Autodesk Fusion 360 part; units mm, degrees
sketch "Sketch1" plane through (0, 0, 0) normal (0, 1, 0) x (1, 0, 0)
  line L0 (7.5, -22.5) -> (-7.5, -22.5)
  line L1 (-7.5, -22.5) -> (-7.5, 22.5)
  line L2 (-7.5, 22.5) -> (7.5, 22.5)
  line L3 (7.5, 22.5) -> (7.5, -22.5)
  line L4 (7.5, -22.5) -> (-7.5, 22.5) construction
  line L5 (-7.5, -22.5) -> (7.5, 22.5) construction
  dimension "d1" = 45
  dimension "d2" = 15
extrude "Extrude1" add sketch "Sketch1" along normal blind 4
sketch "Sketch2" plane through (0, 4, 0) normal (0, 1, 0) x (-1, 0, 0)
  line L0 (-7.5, -22.5) -> (7.5, -22.5)
  line L1 (7.5, -22.5) -> (7.5, 22.5)
  line L2 (7.5, 22.5) -> (-7.5, 22.5)
  line L3 (-7.5, 22.5) -> (-7.5, -22.5)
  line L4 (-7.5, 22.5) -> (-3.5, 22.5)
  line L5 (-3.5, 22.5) -> (-3.5, -22.5)
  line L6 (-3.5, -22.5) -> (-7.5, -22.5)
  line L7 (-7.5, -22.5) -> (-7.5, 22.5)
  dimension "d9" = 4
extrude "Extrude2" add sketch "Sketch2" along normal blind 64 contours L0 L2 L3 L4 L5 L6 L7
sketch "Sketch3" plane through (3.5, 0, 0) normal (-1, 0, 0) x (0, -1, 0)
  line L0 (-4, -22.5) -> (-4, 22.5)
  line L1 (-4, 22.5) -> (-68, 22.5)
  line L2 (-68, 22.5) -> (-68, -22.5)
  line L3 (-68, -22.5) -> (-4, -22.5)
  line L4 (-68, 22.5) -> (-64, 22.5)
  line L5 (-64, 22.5) -> (-64, -22.5)
  line L6 (-64, -22.5) -> (-68, -22.5)
  line L7 (-68, -22.5) -> (-68, 22.5)
  dimension "d12" = 4
extrude "Extrude3" add sketch "Sketch3" along normal blind 11 contours L1 L2 L3 L4 L5 L6 L7
sketch "Sketch4" plane through (3.5, 0, 0) normal (-1, 0, 0) x (0, -1, 0)
  line L0 (-64, 22.5) -> (-64, -22.5)
  line L1 (-64, -22.5) -> (-4, -22.5)
  line L2 (-4, -22.5) -> (-4, 22.5)
  line L3 (-4, 22.5) -> (-64, 22.5)
  line L4 (-60, 22.5) -> (-56, 22.5)
  line L5 (-56, 22.5) -> (-56, -22.5)
  line L6 (-56, -22.5) -> (-60, -22.5)
  line L7 (-60, -22.5) -> (-60, 22.5)
  line L8 (-34, -22.5) -> (-34, 22.5) construction
  line L9 (-8, 22.5) -> (-12, 22.5)
  line L10 (-8, -22.5) -> (-8, 22.5)
  line L11 (-12, 22.5) -> (-12, -22.5)
  line L12 (-12, -22.5) -> (-8, -22.5)
  dimension "d15" = 4
  dimension "d16" = 4
sketch "Sketch5" plane through (0, 68, 0) normal (0, 1, 0) x (-1, 0, 0)
  line L0 (-7.5, -22.5) -> (7.5, -22.5)
  line L1 (7.5, -22.5) -> (7.5, 22.5)
  line L2 (7.5, 22.5) -> (-7.5, 22.5)
  line L3 (-7.5, 22.5) -> (-7.5, -22.5)
  circle A0 centre (3.5, 17.4201) radius 2
  circle A1 centre (3.5, -17.5799) radius 2
  line L4 (3.5, -17.5799) -> (3.5, 17.4201) construction
  point P0 (3.5, -0.0799)
  dimension "d19" = 4
  dimension "d20" = 4
  dimension "d21" = 35
  dimension "d22" = 4
extrude "Extrude5" cut sketch "Sketch5" against normal through all contours A0 | A1
ref_plane "WorkPlane1" through (0, 34, 0) normal (0, 1, 0) x (0, 0, 1)
sketch "Sketch6" plane through (0, 34, 0) normal (0, 1, 0) x (1, 0, 0)
  line L0 (7.5, -12.5) -> (42.8553, -47.8553)
  line L1 (7.5, 22.5) -> (7.5, -22.5)
  line L2 (7.5, 12.5) -> (7.5, -12.5) construction
  line L3 (7.5, 0) -> (0, 0)
  line L4 (42.8553, -47.8553) -> (44.6231, -46.0876)
  line L5 (44.6231, -42.552) -> (7.5, -5.4289)
  arc A0 (44.6231, -46.0876) -> (44.6231, -42.552) centre (42.8553, -44.3198) ccw
  point P0 (7.5, 0)
  point P1 (46.3909, -44.3198)
  dimension "d25" = 50
  dimension "d26" = 25
  dimension "d27" = 135
  dimension "d29" = 5
  dimension "d30" = 2.5
revolve "Revolve1" add sketch "Sketch6" angle 360 about axis through (7.5, 34, 0) along (-1, 0, 0)
equation "d10 = 56 mm + 8 mm"
equation "d24 = -( 68 / 2 ) * 1 mm"
Verification items for the finished model (mm, model axes). A direction names the side the tool comes from. Coordinates: 2 decimals unless noted, no trailing zeros. Order: outer loops, then holes, each group sorted by start corner. A loop starts at its lowest first (then second) coordinate and runs counter-clockwise, first axis right, second up. Notation, with made-up numbers: M -17,48.5 L 35,48.5 A9 cw 35,62.5 Z; hole C 31,-33.75 d4. An arc over 180 degrees is marked long. Write each question's results on one line, items separated by ' | '.
1) Release check for a two-part mould opening along X. For faces 1 (the face through (0, 0, 0)), 2 (the face through (-7.5, 2, 0)), 3 (the face through (-3.066, 2.028, -19.532)) record: pulls with the +X half, pulls with the -X half, needs draft (parallel to the pull), parting line crosses it, or undercut.
Solved:
face 1: needs draft | face 2: pulls with the -X half | face 3: undercut
2) Section check C-C on x = 29. Record the cut outline in (y, z).
Solved:
outline: C 34,0 d68; hole C 34,0 d53.86
3) Scan lines: line 1 along Z through (x, y) = (-3.5, 3.1); line 2 along Z through (x, y) = (-3, 66); line 3 along Z through (x, y) = (38, 16). Record each from-to range of solid material in increasing order. Write a range as [from, to].
Solved:
line 1: z = [-22.5, -19.58], [-15.58, 15.42], [19.42, 22.5] | line 2: z = [-22.5, -19.52], [-15.64, 15.48], [19.36, 22.5] | line 3: z = [-39.05, -31.09], [31.09, 39.05]
4) Section check D-D on x = 14. Record the cut outline in (y, z).
Solved:
outline: C 34,0 d38; hole C 34,0 d23.86
5) Section check B-B on z = 0. Record the cut outline in (x, y), plus the area to 3 significant figures.
Solved:
outline: M -7.5,0 L 7.5,0 L 7.5,21.5 L 42.86,-13.86 L 44.62,-12.09 A2.5 ccw 44.62,-8.55 L 7.5,28.57 L 7.5,39.43 L 44.62,76.55 A2.5 ccw 44.62,80.09 L 42.86,81.86 L 7.5,46.5 L 7.5,68 L -7.5,68 L -7.5,64 L 3.5,64 L 3.5,4 L -7.5,4 Z | area: 882 mm²
6) Gauge pin test, flat ends, axial feed: pin 1 Ø4 at (y, z) = (50.5, 23) entering from -X; pin 2 Ø12 at (x, z) = (0, -6) entering from +Y; pin 3 Ø12 at (x, y) = (17, 8.5) entering from -Z. Record the tip position at first contact, or that the pin passes through.
Solved:
pin 1: stops at x = 3.5 | pin 2: stops at y = 68 | pin 3: stops at z = -15.46
7) Access from +Z, -Z, +X, -X, +Y, -Y to the whole of each face (thin tool, end or side, straight path). Record for faces 4 (the face through (4, 34, 22.5)), 5 (the face through (7.5, 34, 0)), 6 (the face through (3.5, 34, 0)).
Solved:
face 4: +Z, -X, +Y, -Y | face 5: +X | face 6: +Z, -Z, -X
8) Section check A-A on x = 0. Record the cut outline in (y, z), plus the area to 3 significant figures.
Solved:
outline: M 0,-22.5 L 4,-22.5 L 4,22.5 L 0,22.5 Z; M 64,-22.5 L 68,-22.5 L 68,22.5 L 64,22.5 Z | area: 360 mm²
